Build history of the part. All positions in model axes, mm. Face numbers are marked on the shaded views. A direction names the side the tool comes from. Round coordinates to 2 decimals unless told otherwise and drop trailing zeros. Write each loop counter-clockwise with the first axis right and the second up, starting at its lowest first coordinate (ties: lowest second). Pieces come first, ordered by that corner, then holes. Notation, with made-up numbers: M 54,85.25 L 76,85.25 A14 ccw 76,97.25 Z; hole C -27.75,-28.5 d5. An arc over 180 degrees is marked long. Use a Markdown table: item, result.
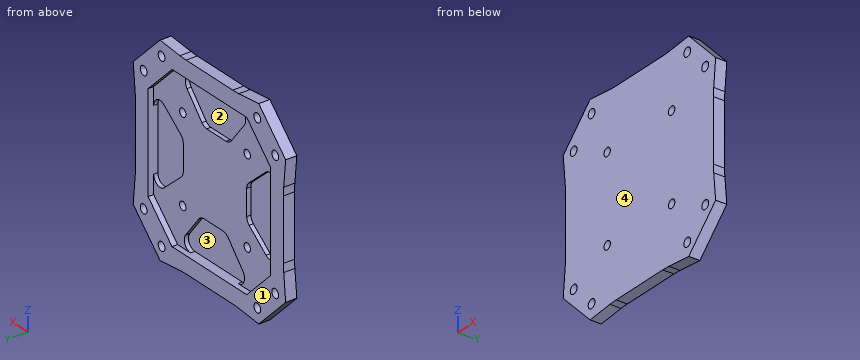
from build123d import *

# Parameters (mm, degrees)
SKETCH1_R           = 1.6
BOSS_EXTRUDE1_DEPTH = 4
CUT_EXTRUDE1_DEPTH  = 2
CUT_EXTRUDE2_DEPTH  = 1.5
SKETCH5_R           = 1.5
CUT_EXTRUDE3_DEPTH  = 52.039025935
FILLET1_R           = 30


with BuildPart() as part:
    # Sketch1 → Boss-Extrude1 (new body)
    with BuildSketch(Plane(origin=(0, 0, 0), x_dir=(1, 0, 0), z_dir=(0, 1, 0))):
        Polygon((-35, 12.5), (-36.062322224, 23.334400163), (-23.334400163, 36.062322224), (-12.5, 35), (12.5, 35), (23.334400163, 36.062322224), (36.062322224, 23.334400163), (35, 12.5), (35, -12.5), (36.062322224, -23.334400163), (23.334400163, -36.062322224), (12.5, -35), (-12.5, -35), (-23.334400163, -36.062322224), (-36.062322224, -23.334400163), (-35, -12.5), align=None)
        with Locations(Location((31.112574756, 22.627293382, 0), (0, 0, 270))):
            Circle(SKETCH1_R, mode=Mode.SUBTRACT)
        with Locations(Location((22.627293382, 31.112574756, 0), (0, 0, 270))):
            Circle(SKETCH1_R, mode=Mode.SUBTRACT)
        with Locations(Location((31.112574756, -22.627293382, 0), (0, 0, 270))):
            Circle(SKETCH1_R, mode=Mode.SUBTRACT)
        with Locations(Location((22.627293382, -31.112574756, 0), (0, 0, 270))):
            Circle(SKETCH1_R, mode=Mode.SUBTRACT)
        with Locations(Location((-22.627293382, -31.112574756, 0), (0, 0, 270))):
            Circle(SKETCH1_R, mode=Mode.SUBTRACT)
        with Locations(Location((-31.112574756, -22.627293382, 0), (0, 0, 270))):
            Circle(SKETCH1_R, mode=Mode.SUBTRACT)
        with Locations(Location((-31.112574756, 22.627293382, 0), (0, 0, 270))):
            Circle(SKETCH1_R, mode=Mode.SUBTRACT)
        with Locations(Location((-22.627293382, 31.112574756, 0), (0, 0, 270))):
            Circle(SKETCH1_R, mode=Mode.SUBTRACT)
    extrude(amount=BOSS_EXTRUDE1_DEPTH)

    # Sketch3 → Cut-Extrude1 (cut)
    with BuildSketch(Plane(origin=(0, 4, 0), x_dir=(1, 0, 0), z_dir=(0, 1, 0))):
        Polygon((-17.668800325, 29), (17.668800325, 29), (29, 17.668800325), (29, -17.668800325), (17.668800325, -29), (-17.668800325, -29), (-29, -17.668800325), (-29, 17.668800325), align=None)
    extrude(amount=-CUT_EXTRUDE1_DEPTH, mode=Mode.SUBTRACT)

    # Sketch4 → Cut-Extrude2 (cut)
    with BuildSketch(Plane(origin=(0, 2, 0), x_dir=(1, 0, 0), z_dir=(0, 1, 0))):
        with BuildLine():
            Line((-29, -11.00200097), (-29, 11.520078787))
            ThreePointArc((-29, 11.520078787), (-27.315491792, 14.216276359), (-24.153679103, 13.884629304))
            Line((-24.153679103, 13.884629304), (-16.153679103, 7.637959136))
            ThreePointArc((-16.153679103, 7.637959136), (-15.303802428, 6.588900412), (-15, 5.273408619))
            Line((-15, 5.273408619), (-15, -3.912899337))
            ThreePointArc((-15, -3.912899337), (-15.264226315, -5.143972993), (-16.010361564, -6.158191945))
            Line((-16.010361564, -6.158191945), (-24.010361564, -13.247293577))
            ThreePointArc((-24.010361564, -13.247293577), (-27.231073656, -13.737774655), (-29, -11.00200097))
        make_face()
        with BuildLine():
            Line((13.884629304, 24.153679103), (7.637959136, 16.153679103))
            ThreePointArc((7.637959136, 16.153679103), (6.588900412, 15.303802428), (5.273408619, 15))
            Line((5.273408619, 15), (-3.912899337, 15))
            ThreePointArc((-3.912899337, 15), (-5.143972993, 15.264226315), (-6.158191945, 16.010361564))
            Line((-6.158191945, 16.010361564), (-13.247293578, 24.010361564))
            ThreePointArc((-13.247293578, 24.010361564), (-13.737774655, 27.231073656), (-11.00200097, 29))
            Line((-11.00200097, 29), (11.520078787, 29))
            ThreePointArc((11.520078787, 29), (14.216276359, 27.315491792), (13.884629304, 24.153679103))
        make_face()
        with BuildLine():
            Line((24.153679103, -13.884629304), (16.153679103, -7.637959136))
            ThreePointArc((16.153679103, -7.637959136), (15.303802428, -6.588900412), (15, -5.273408619))
            Line((15, -5.273408619), (15, 3.912899337))
            ThreePointArc((15, 3.912899337), (15.264226315, 5.143972993), (16.010361564, 6.158191945))
            Line((16.010361564, 6.158191945), (24.010361564, 13.247293578))
            ThreePointArc((24.010361564, 13.247293578), (27.231073656, 13.737774655), (29, 11.00200097))
            Line((29, 11.00200097), (29, -11.520078787))
            ThreePointArc((29, -11.520078787), (27.315491792, -14.216276359), (24.153679103, -13.884629304))
        make_face()
        with BuildLine():
            Line((-13.884629304, -24.153679103), (-7.637959136, -16.153679103))
            ThreePointArc((-7.637959136, -16.153679103), (-6.588900412, -15.303802428), (-5.273408619, -15))
            Line((-5.273408619, -15), (3.912899337, -15))
            ThreePointArc((3.912899337, -15), (5.143972993, -15.264226315), (6.158191945, -16.010361564))
            Line((6.158191945, -16.010361564), (13.247293578, -24.010361564))
            ThreePointArc((13.247293578, -24.010361564), (13.737774655, -27.231073656), (11.00200097, -29))
            Line((11.00200097, -29), (-11.520078787, -29))
            ThreePointArc((-11.520078787, -29), (-14.216276359, -27.315491792), (-13.884629304, -24.153679103))
        make_face()
    extrude(amount=-CUT_EXTRUDE2_DEPTH, mode=Mode.SUBTRACT)

    # Sketch5 → Cut-Extrude3 (cut, through all)
    with BuildSketch(Plane(origin=(0, 2, 0), x_dir=(1, 0, 0), z_dir=(0, 1, 0))):
        with Locations(Location((15.25, 15.25, 0), (0, 0, 270))):
            Circle(SKETCH5_R)
        with Locations(Location((15.25, -15.25, 0), (0, 0, 270))):
            Circle(SKETCH5_R)
        with Locations(Location((-15.25, -15.25, 0), (0, 0, 270))):
            Circle(SKETCH5_R)
        with Locations(Location((-15.25, 15.25, 0), (0, 0, 270))):
            Circle(SKETCH5_R)
    extrude(amount=-CUT_EXTRUDE3_DEPTH, mode=Mode.SUBTRACT)

    # Fillet1
    # the kernel refuses this fillet: 30 mm, written as the material it adds along each edge
    with BuildSketch(Plane(origin=(-35, 0, -12.5), x_dir=(-0.09758289975914561, 0, -0.9952273999818315), z_dir=(0, 1, 0)), Plane(origin=(12.5, 0, 35), x_dir=(-1, 0, 0), z_dir=(0, 1, 0)), Plane(origin=(-12.5, 0, 35), x_dir=(-0.9952273999818316, 0, 0.09758289975914514), z_dir=(0, 1, 0)), Plane(origin=(-35, 0, 12.5), x_dir=(0, 0, -1), z_dir=(0, 1, 0))) as fillet1_piece_1:
        with BuildLine():
            CenterArc((FILLET1_R * 0.0489081594208, FILLET1_R), FILLET1_R, 264.4, 5.6)
            Line((-FILLET1_R * 0.0486747403383, FILLET1_R * 0.00477260001817), (0, 0))
            Line((0, 0), (FILLET1_R * 0.0489081594208, 0))
        make_face()
    extrude(amount=4)
    with BuildSketch(Plane(origin=(-12.5, 0, -35), x_dir=(-0.9952273999818313, 0, -0.09758289975914779), z_dir=(0, 1, 0)), Plane(origin=(12.5, 0, -35), x_dir=(-1, 0, 0), z_dir=(0, 1, 0)), Plane(origin=(35, 0, -12.5), x_dir=(0.0975828997591479, 0, -0.9952273999818313), z_dir=(0, 1, 0)), Plane(origin=(35, 0, 12.5), x_dir=(0, 0, -1), z_dir=(0, 1, 0))) as fillet1_piece_2:
        with BuildLine():
            CenterArc((FILLET1_R * 0.0489081594208, -FILLET1_R), FILLET1_R, 90, 5.6)
            Line((-FILLET1_R * 0.0486747403383, -FILLET1_R * 0.00477260001817), (0, 0))
            Line((0, 0), (FILLET1_R * 0.0489081594208, 0))
        make_face()
    extrude(amount=4)


solid = part.part
Q1. Cut at B-B on y = 2.75. Count the separate pieces of the cut face and the enclosed holes in it, and give its area (3 significant figures).
Response values:
| item | result |
|---|---|
| separate pieces | 1 |
| enclosed holes | 9 |
| area | 1,550 mm2 |
Q2. Cut at A-A on x = 3. Give the cut face in (y, z).
Response values:
| item | result |
|---|---|
| outline | M 0,-35 L 4,-35 L 4,-29 L 0.5,-29 L 0.5,-15 L 2,-15 L 2,15 L 0.5,15 L 0.5,29 L 4,29 L 4,35 L 0,35 Z |
Q3. Two-plate mould, pull along Z, no slides. Class the marked faces 1 and 2: +Z half, -Z half, draft (parallel to the pull), parting line (faces both ways), or undercut.
Response values:
| item | result |
|---|---|
| face 1 | draft |
| face 2 | undercut |
Q4. Drop flat-ended pins along their axis: P1, Ø4, axis at x = 15.25, z = -15.25, coming from the +Y side; P2, Ø1.6, axis at y = 1, z = -1, coming from the -X side; P3, Ø1, axis at y = 2.5, z = 3.5, coming from the +X side. Give the stop position or say it passes through.
Response values:
| item | result |
|---|---|
| P1 | stops at y = 2 |
| P2 | stops at x = -35 |
| P3 | stops at x = 35 |
Q5. Drill centre lines: L1, parallel to X at y = 0.6, z = 3; L2, parallel to Z at x = 9, y = 0.8; L3, parallel to Z at x = 13, y = 1.15. Where is each one in solid material? Low to high.
Response values:
| item | result |
|---|---|
| L1 | x = -35 to -29, -15 to 15, 29 to 35 |
| L2 | z = -35 to -29, -17.9 to 19.22, 29 to 35 |
| L3 | z = -35.06 to -28.61, -23.02 to 23.73, 28.24 to 35.06 |
Q6. Which spindle directions (+Z, -Z, +X, -X, +Y, -Y) get a long thin tool onto all of the face, cutting with end or side? Do the marked faces 3 and 4. Say none if no direction does.
Response values:
| item | result |
|---|---|
| face 3 | +Y |
| face 4 | +Z, -Z, +X, -X, -Y |
